Input: part model. Units: mm. Frame: model coordinates. A direction names the side the tool comes from. Coordinates: 2 decimals unless noted, no trailing zeros. Loops run counter-clockwise (first coordinate to the right, second up) from the corner with the lowest first, then second, coordinate; pieces in that order, holes last. Notation, with made-up numbers: (60.25, 55.5) - (76.25, 55.5) arc R25 ccw to (76.25, 81.5) - close; hole circle Ø7 at (-5, 67). An arc over 180 degrees is marked (long way). Answer as CSV lines item,"result". Start each with the question number.
```python
from build123d import *

# Parameters (mm, degrees)
EXTRUDE_1_DEPTH = 5
EXTRUDE_2_DEPTH = 7.5


with BuildPart() as part:
    # 草图1 → 凸台-拉伸1 (new body)
    with BuildSketch(Plane.XY):
        Polygon((-101.128293069, 0), (-86.128293069, 9), (-86.128293069, 21), (-98.628293069, 21), (-98.628293069, 34), (-58.628293069, 34), (-71.128293069, 21), (-71.128293069, 9), (-56.128293069, 0), align=None)
    extrude(amount=EXTRUDE_1_DEPTH)

    # 草图2 → 凸台-拉伸2 (add)
    with BuildSketch(Plane(origin=(0, 0, 5), x_dir=(-1, 0, 0), z_dir=(0, 0, -1))):
        Polygon((54.8921871, 35), (70.128293069, 19.154449793), (70.128293069, 10.732380758), (56.128293069, 2.332380758), (56.128293069, 0), (71.128293069, 9), (71.128293069, 21), (58.628293069, 34), (98.628293069, 34), (98.628293069, 21), (86.128293069, 21), (86.128293069, 9), (101.128293069, 0), (101.128293069, 2.332380758), (87.128293069, 10.732380758), (87.128293069, 20), (100.628293069, 20), (100.628293069, 29), (100.628293069, 35), align=None)
    extrude(amount=EXTRUDE_2_DEPTH)


solid = part.part
```
Item 1: Section query C-C, the plane y = 32.5. Output: boundary loops of the cut face in (x, z), and give its area (3 significant figures).
Item 2: Set-up query: faces 5 (the flat face through (-78, 34, -1)), 6 (the flat face through (-71.128, 15, -1)), 7 (the flat face through (-70.128, 15, 1)), 8 (the flat face through (-100.628, 27, 1)), 9 (the flat face through (-78, 0, 2)). Return all of +Z, -Z, +X, -X, +Y, -Y with unobstructed straight access to the full face (end or side cutting, diameter ignored); none if empty.
Item 3: Draft query along X for faces 1 (the flat face through (-63.523, 4.437, -1.232)), 2 (the flat face through (-98.628, 28, -1)), 3 (the flat face through (-94, 20, 1)), 4 (the flat face through (-94.23, 6.47, 1.3)). Return one class per face: pulls with the +X half, pulls with the -X half, needs draft (parallel to the pull), parting line crosses it, or undercut.
Item 4: Section query D-D, the plane x = -85. Output: boundary loops of the cut face in (y, z), and give its area (4 significant figures).
Item 5: Material intervals for probe 1 along X at (y, z) = (15, -0.5); probe 2 along X at (y, z) = (2, 4); probe 3 along X at (y, z) = (11.5, 2.5), sorted ascending.
Item 6: Section query A-A, the plane x = -58. Output: boundary loops of the cut face in (y, z).
Item 7: Contact query for flat-ended pins moving along their axis: P1, Ø1, axis at x = -72.5, y = 26.5, coming from the -Z side; P2, Ø2, axis at x = -84, z = -1.5, coming from the -Y side; P3, Ø1.9, axis at y = 1, z = 2, coming from the +X side; P4, Ø4, axis at x = -94, z = 1.5, coming from the -Y side. Output: stop coordinate, or through.
Item 8: Section query B-B, the plane z = 1.5. Output: boundary loops of the cut face in (x, y).
Response values:
1,outline,"(-100.63, -2.5) - (-98.63, -2.5) - (-98.63, 0) - (-60.07, 0) - (-60.07, -2.5) - (-57.3, -2.5) - (-57.3, 5) - (-100.63, 5) - close"
1,area,"229 mm²"
2,face 5,"-Z"
2,face 6,"-Z, -Y"
2,face 7,"+Z, -Z, +X"
2,face 8,"+Z, -Z, -X, +Y"
2,face 9,"+Z, -Z, +X, -X, -Y"
3,face 1,"undercut"
3,face 2,"undercut"
3,face 3,"needs draft"
3,face 4,"pulls with the -X half"
4,outline,"(0, 0) - (34, 0) - (34, -2.5) - (35, -2.5) - (35, 5) - (0, 5) - close"
4,area,"177.5 mm²"
5,probe 1,"x = -87.13 to -86.13, -71.13 to -70.13"
5,probe 2,"x = -101.13 to -56.13"
5,probe 3,"x = -87.13 to -70.13"
6,outline,"(0, 0) - (1.12, 0) - (1.12, -2.5) - (3.46, -2.5) - (3.46, 5) - (0, 5) - close; (31.77, -2.5) - (35, -2.5) - (35, 5) - (31.77, 5) - close"
7,P1,"stops at z = 0"
7,P2,"stops at y = 34"
7,P3,"stops at x = -56.13"
7,P4,"stops at y = 0"
8,outline,"(-101.13, 0) - (-56.13, 0) - (-56.13, 2.33) - (-70.13, 10.73) - (-70.13, 19.15) - (-54.89, 35) - (-100.63, 35) - (-100.63, 20) - (-87.13, 20) - (-87.13, 10.73) - (-101.13, 2.33) - close"
